Autodesk Fusion 360 part; units mm, degrees
sketch "Sketch1" plane through (0, 0, 0) normal (0, 0, 1) x (1, 0, 0)
  line L0 (-90, 90) -> (90, 90)
  line L1 (90, 90) -> (90, -90)
  line L2 (90, -90) -> (-90, -90)
  line L3 (-90, -90) -> (-90, 90)
  line L4 (-90, 90) -> (90, -90) construction
  line L5 (90, 90) -> (-90, -90) construction
  dimension "d1" = 180
  dimension "d2" = 180
extrude "Extrude1" add sketch "Sketch1" along normal blind 10
sketch "Sketch2" plane through (0, 0, 10) normal (0, 0, 1) x (-1, 0, 0)
  line L0 (90, 90) -> (-90, 90)
  line L1 (-90, 90) -> (-90, -90)
  line L2 (-90, -90) -> (90, -90)
  line L3 (90, -90) -> (90, 90)
  circle A0 centre (0, 0) radius 70
  dimension "d5" = 140
extrude "Extrude2" add sketch "Sketch2" along normal blind 100 contours A0
sketch "Sketch3" plane through (0, 0, 0) normal (0, 1, 0) x (1, 0, 0)
  line L0 (-40, -80) -> (40, -80)
  line L1 (40, -80) -> (40, -40)
  line L2 (40, -40) -> (-40, -40)
  line L3 (-40, -40) -> (-40, -80)
  line L4 (-40, -80) -> (40, -40) construction
  line L5 (40, -80) -> (-40, -40) construction
  point P0 (0, -60)
  dimension "d13" = 40
  dimension "d14" = 80
  dimension "d16" = 60
extrude "Extrude3" add sketch "Sketch3" against normal blind 100
sketch "Sketch4" plane through (0, 0, 110) normal (0, 0, 1) x (-1, 0, 0)
  circle A0 centre (0, 0) radius 70
  circle A1 centre (0, 0) radius 65
  dimension "d10" = -5
extrude "Extrude4" cut sketch "Sketch4" against normal blind 10 contours A1
extrude "Extrude5" add 1 faces at (2.3225, -16.9397, 100) along direction (0, 0, 1) blind 7
sketch "Sketch5" plane through (0, 0, 10) normal (0, 0, 1) x (-1, 0, 0)
  circle A0 centre (0, 0) radius 70
  line L0 (90, 90) -> (-90, 90)
  line L1 (-90, 90) -> (-90, -90)
  line L2 (-90, -90) -> (90, -90)
  line L3 (90, -90) -> (90, 90)
  point P0 (80, -80)
  point P1 (-80, -80)
  point P2 (-80, 80)
  point P3 (80, 80)
  point P4 (116.0582, 65.2033)
  dimension "d19" = 10
  dimension "d20" = 10
  dimension "d21" = 10
  dimension "d22" = 10
  dimension "d23" = 10
  dimension "d24" = 10
  dimension "d25" = 10
  dimension "d26" = 10
hole "Hole1" at (-80, -80, 10) at (80, -80, 10) at (80, 80, 10) at (-80, 80, 10) direction (0, 0, -1) diameter 7 depth 15 tip angle 118 counterbore diameter 12 counterbore depth 2
fillet "Fillet1" radius 10 8 edges at (-90, -90, 5) (90, -90, 5) (90, 90, 5) (-90, 90, 5) (40, -78.7228, 80) (40, -78.7228, 40) (-40, -78.7228, 80) (-40, -78.7228, 40)
fillet "Fillet2" radius 2 24 edges at (87.0711, -87.0711, 10) (90, 0, 10) (87.0711, 87.0711, 10) (0, 90, 10) (-87.0711, 87.0711, 10) (-90, 0, 10) (-87.0711, -87.0711, 10) (0, -90, 10) (-37.0711, -100, 77.0711) (-40, -100, 60) (-37.0711, -100, 42.9289) (0, -100, 40) (37.0711, -100, 42.9289) (40, -100, 60) (37.0711, -100, 77.0711) (0, -100, 80) (36.9012, -59.4835, 77.2363) (40, -57.4456, 60) (36.9012, -59.4835, 42.7637) (0, -70, 40) (-36.9012, -59.4835, 42.7637) (-40, -57.4456, 60) (-36.9012, -59.4835, 77.2363) (0, -70, 80)
Geometry: final body of the model. Coordinates: model frame, mm. A direction names the side the tool comes from. Coordinates: 2 decimals unless noted, no trailing zeros. Order: outer loops, then holes, each group sorted by start corner. A loop starts at its lowest first (then second) coordinate and runs counter-clockwise, first axis right, second up.
(1) Material intervals for probe 1 along Y at (x, z) = (-80, 2); probe 2 along Y at (x, z) = (80, 9), sorted ascending.
(2) Section query D-D (y = -19). Return the cut outline in (x, z), plus the area to 3 significant figures.
(3) Section query C-C (z = 99.5). Return the cut outline in (x, y).
(4) Draft query along Z for faces 1 (the face through (-1, 90, 4)), 2 (the face through (-36.99, -78.52, 77.15)), 3 (the face through (36.99, -78.52, 42.85)). Return one class per face: pulls with the +Z half, pulls with the -Z half, needs draft (parallel to the pull), parting line crosses it, or undercut.
(5) Access query for faces 4 (the face through (-37.15, -78.52, 43.01)), 5 (the face through (-77, -83, 8)), 6 (the face through (-61.9, 20.4, 110)). Directions: +Z, -Z, +X, -X, +Y, -Y. A direction counts if a zero-diameter tool reaches every point of the face in a straight line with its end or side. Return the directions, or none.
(6) First-contact query: pin 1 (10 mm diameter, centred on x = -8, y = -77, fed in from +Z); pin 2 (12 mm diameter, centred on x = 0.5, y = 24, fed in from -Z); pin 3 (12 mm diameter, centred on y = -37.5, z = 71, fed in from -X); pin 4 (22 mm diameter, centred on y = -80.5, z = 63, fed in from +X). Flat tips, straight axial feed; report the tip coordinate or a pass-through.
(7) Section query A-A (y = 0). Return the cut outline in (x, z).
(8) Section query B-B (x = 0). Return the cut outline in (y, z).
Solution:
1. probe 1: y = -90 to -83.5, -76.5 to 76.5, 83.5 to 90
1. probe 2: y = -89.73 to -86, -74 to 74, 86 to 89.73
2. outline: (-90, 0) - (90, 0) - (90, 8) arc R2 ccw to (88, 10) - (67.37, 10) - (67.37, 110) - (62.16, 110) - (62.16, 107) - (-62.16, 107) - (-62.16, 110) - (-67.37, 110) - (-67.37, 10) - (-88, 10) arc R2 ccw to (-90, 8) - close
2. area: 14,900 mm2
3. outline: circle Ø140 at (0, 0)
4. face 1: needs draft
4. face 2: pulls with the +Z half
4. face 3: undercut
5. face 4: -X, -Y
5. face 5: +Z
5. face 6: +Z, +X, -X, +Y, -Y
6. pin 1: stops at z = 80
6. pin 2: stops at z = 0
6. pin 3: stops at x = -62.51
6. pin 4: stops at x = 40
7. outline: (-90, 0) - (90, 0) - (90, 8) arc R2 ccw to (88, 10) - (70, 10) - (70, 110) - (65, 110) - (65, 107) - (-65, 107) - (-65, 110) - (-70, 110) - (-70, 10) - (-88, 10) arc R2 ccw to (-90, 8) - close
8. outline: (-100, 42) arc R2 ccw to (-98, 40) - (-72, 40) arc R2 cw to (-70, 38) - (-70, 10) - (-88, 10) arc R2 ccw to (-90, 8) - (-90, 0) - (90, 0) - (90, 8) arc R2 ccw to (88, 10) - (70, 10) - (70, 110) - (65, 110) - (65, 107) - (-65, 107) - (-65, 110) - (-70, 110) - (-70, 82) arc R2 cw to (-72, 80) - (-98, 80) arc R2 ccw to (-100, 78) - close
